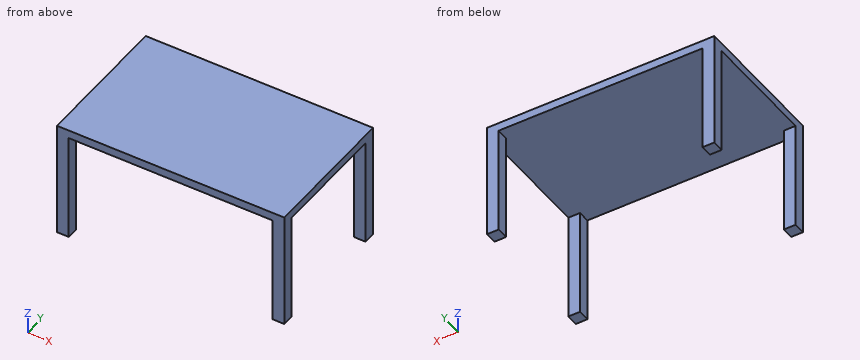
from build123d import *

# Parameters (mm, degrees)
F0_W     = 70
F0_H     = 70
F1_DEPTH = 650
F2_START = 650
F2_DEPTH = 50


with BuildPart() as f1:
    # F0 (on Top) → F1 (new body)
    with BuildSketch(Plane.XY):
        with Locations((-645, 385)):
            Rectangle(F0_W, F0_H)
    extrude(amount=F1_DEPTH)



with BuildPart() as f1b:
    # F0 (on Top) → F1, piece 2 (new body)
    with BuildSketch(Plane.XY):
        with Locations((645, 385)):
            Rectangle(F0_W, F0_H)
    extrude(amount=F1_DEPTH)


with BuildPart() as f1c:
    # F0 (on Top) → F1, piece 3 (new body)
    with BuildSketch(Plane.XY):
        with Locations((645, -385)):
            Rectangle(F0_W, F0_H)
    extrude(amount=F1_DEPTH)


with BuildPart() as f1d:
    # F0 (on Top) → F1, piece 4 (new body)
    with BuildSketch(Plane.XY):
        with Locations((-645, -385)):
            Rectangle(F0_W, F0_H)
    extrude(amount=F1_DEPTH)


with BuildPart() as f1_1:
    add(f1.part)

    add(f1b.part)  # F2 merges F1b

    add(f1c.part)  # F2 merges F1c

    add(f1d.part)  # F2 merges F1d
    # F0 (on Top) → F2 (join)
    with BuildSketch(Plane.XY.offset(F2_START)):
        with Locations((-645, 385)):
            Rectangle(F0_W, F0_H)
        Polygon((610, 420), (-610, 420), (-610, 350), (-680, 350), (-680, -350), (-610, -350), (-610, -420), (610, -420), (610, -350), (680, -350), (680, 350), (610, 350), align=None)
        with Locations((-645, -385)):
            Rectangle(F0_W, F0_H)
        with Locations((645, 385)):
            Rectangle(F0_W, F0_H)
        with Locations((645, -385)):
            Rectangle(F0_W, F0_H)
    extrude(amount=F2_DEPTH)


solid = f1_1.part
The model under review builds one solid part; all positions refer to its coordinate system, in mm. Coordinates: 2 decimals unless noted, no trailing zeros. Loops run counter-clockwise (first coordinate to the right, second up) from the corner with the lowest first, then second, coordinate; pieces in that order, holes last.
(1) Wall thickness on L1, parallel to X at y = -351, z = 322; L2, parallel to Z at x = 105, y = 4: over which ranges is each line inside the solid? List them lowest first.
Determined:
L1: x = -680 to -610, 610 to 680
L2: z = 650 to 700
(2) Consider section C-C, the plane y = -23. Give the boundary of the cut face in (x, z).
Determined:
outline: (-680, 650) - (680, 650) - (680, 700) - (-680, 700) - close
(3) Insertion check: P1, Ø1.5, axis at x = -384.5, y = 312.5, coming from the -Z side. The pin has a flat end and moves straight along its axis. Give the tip position at first contact, or say it passes through.
Determined:
P1: stops at z = 650
(4) Consider section A-A, the plane z = 146. Give the boundary of the cut face in (x, y).
Determined:
outline: (-680, -420) - (-610, -420) - (-610, -350) - (-680, -350) - close; (-680, 350) - (-610, 350) - (-610, 420) - (-680, 420) - close; (610, -420) - (680, -420) - (680, -350) - (610, -350) - close; (610, 350) - (680, 350) - (680, 420) - (610, 420) - close
(5) Consider section B-B, the plane x = 537. Give the boundary of the cut face in (y, z).
Determined:
outline: (-420, 650) - (420, 650) - (420, 700) - (-420, 700) - close
